```python
from build123d import *

# Parameters (mm, degrees)
SKETCH1_R                                       = 9
BOSS_EXTRUDE1_DEPTH                             = 10
SKETCH2_R                                       = 3
CUT_EXTRUDE1_DEPTH                              = 96.94790253
BOSS_EXTRUDE2_DEPTH                             = 3
SKETCH3_W                                       = 4
SKETCH3_H                                       = 8
CUT_EXTRUDE2_DEPTH                              = 97.695398029
RIB4_REACH                                      = 98.695
SKETCH5_WALL_W                                  = 220.579405852
SKETCH5_WALL_H                                  = 10
FILLET1_R                                       = 2
FILLET1_OF_MIRROR1_R                            = 2
SKETCH7_R                                       = 5
CUT_EXTRUDE3_DEPTH                              = 97.695398153
CHAMFER1_SIZE                                   = 1
CSK_FOR_M3_FLAT_HEAD_MACHINE_SCREW1_D           = 3.2
CSK_FOR_M3_FLAT_HEAD_MACHINE_SCREW1_CSINK_D     = 6.3
CSK_FOR_M3_FLAT_HEAD_MACHINE_SCREW1_CSINK_ANGLE = 90


with BuildPart() as part:
    # Sketch1 → Boss-Extrude1 (new body)
    with BuildSketch(Plane.XY):
        Circle(SKETCH1_R)
        with BuildLine():
            ThreePointArc((9, 0), (6.363961031, -6.363961031), (0, -9))
            Line((0, -9), (95, -9))
            Line((95, -9), (95, 7))
            Line((95, 7), (5.656854249, 7))
            ThreePointArc((5.656854249, 7), (8.121320344, 3.878679656), (9, 0))
        make_face()
    extrude(amount=BOSS_EXTRUDE1_DEPTH)

    # Sketch2 → Cut-Extrude1 (cut, through all)
    with BuildSketch(Plane.XY):
        Circle(SKETCH2_R)
    extrude(amount=CUT_EXTRUDE1_DEPTH, mode=Mode.SUBTRACT)

    # Sketch4 → Boss-Extrude2 (add)
    with BuildSketch(Plane(origin=(95, 0, 0), x_dir=(0, 0, -1), z_dir=(1, 0, 0))):
        with BuildLine():
            ThreePointArc((0, -14.076696831), (-5, -15), (-10, -14.076696831))
            Line((-10, -14.076696831), (-10, 12.076696831))
            ThreePointArc((-10, 12.076696831), (-5, 13), (0, 12.076696831))
            Line((0, 12.076696831), (0, -14.076696831))
        make_face()
    extrude(amount=-BOSS_EXTRUDE2_DEPTH)

    # Sketch3 → Cut-Extrude2 (cut, through all)
    with BuildSketch(Plane.XY):
        with Locations((93, -1)):
            Rectangle(SKETCH3_W, SKETCH3_H)
    extrude(amount=CUT_EXTRUDE2_DEPTH, mode=Mode.SUBTRACT)

    # Sketch5 wall → Rib4 (add, up to next)
    with BuildSketch(Plane(origin=(79.5, 8.538348415, 10), x_dir=(-0.992512099864, -0.122146353295, 0), z_dir=(0.122146353295, -0.992512099864, 0)), mode=Mode.PRIVATE) as rib4_sk1:
        with Locations((0, 5)):
            Rectangle(SKETCH5_WALL_W, SKETCH5_WALL_H)
    rib4_tool1 = extrude(rib4_sk1.sketch, amount=RIB4_REACH, mode=Mode.PRIVATE) - part.part
    rib4 = rib4_tool1.solids().sort_by_distance((79.5, 8.538348415, 10))[0]
    add(rib4)

    # Fillet1
    fillet1_edges = [part.edges().sort_by_distance(p)[0] for p in [
        (92, 11.076696831, 0),
        (92, 11.076696831, 10),
        (92, 10.07669683, 5),
        (79.500000002, 8.538348415, 0),
        (79.500000002, 8.538348415, 10),
    ]]
    fillet(fillet1_edges, radius=FILLET1_R)

    # Mirror1: Rib4 across plane
    add(rib4.mirror(Plane.ZX.offset(-1)))

    # Fillet1 of Mirror1
    fillet1_of_mirror1_edges = [part.edges().sort_by_distance(p)[0] for p in [
        (92, -13.076696831, 0),
        (92, -13.076696831, 10),
        (92, -12.07669683, 5),
        (79.500000002, -10.538348415, 0),
        (79.500000002, -10.538348415, 10),
    ]]
    fillet(fillet1_of_mirror1_edges, radius=FILLET1_OF_MIRROR1_R)

    # Sketch7 → Cut-Extrude3 (cut, through all)
    with BuildSketch(Plane.XY):
        with Locations((79.294775575, -1)):
            Circle(SKETCH7_R)
    extrude(amount=CUT_EXTRUDE3_DEPTH, mode=Mode.SUBTRACT)

    # Chamfer1
    chamfer1_edges = [part.edges().sort_by_distance(p)[0] for p in [
        (74.294775575, -1, 0),
        (74.294775575, -1, 10),
    ]]
    chamfer(chamfer1_edges, length=CHAMFER1_SIZE)

    # CSK for M3 Flat Head Machine Screw1 (through all)
    with Locations(Plane(origin=(0, 0, 0), x_dir=(-1, 0, 0), z_dir=(0, 0, -1))):
        with Locations((-17, -6)):
            CounterSinkHole(CSK_FOR_M3_FLAT_HEAD_MACHINE_SCREW1_D / 2, CSK_FOR_M3_FLAT_HEAD_MACHINE_SCREW1_CSINK_D / 2, counter_sink_angle=CSK_FOR_M3_FLAT_HEAD_MACHINE_SCREW1_CSINK_ANGLE)


solid = part.part
```
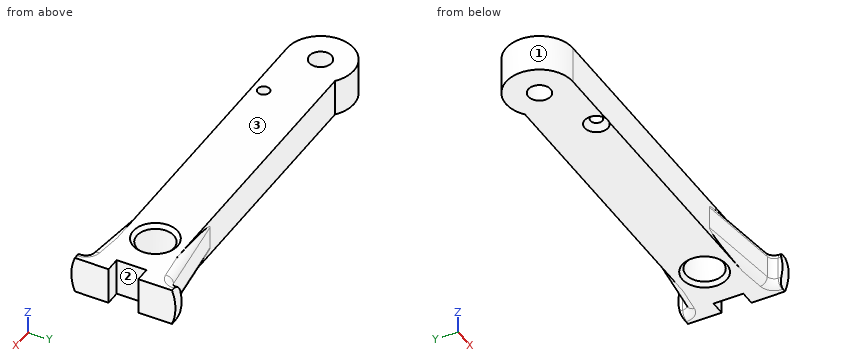
The model under review builds one solid part; all positions refer to its coordinate system, in mm. Face numbers are marked on the shaded views. Coordinates: 2 decimals unless noted, no trailing zeros. Write each loop counter-clockwise with the first axis right and the second up, starting at its lowest first coordinate (ties: lowest second). Pieces come first, ordered by that corner, then holes. Notation, with made-up numbers: (-28.5, 30.25) -> (-4.5, 30.25) arc R31 ccw to (-4.5, 62.25) -> close; hole circle Ø3 at (1, -27.5). An arc over 180 degrees is marked (long way). One line per item, written item: value. Start each with the question number.
Q1. To check wall thickness, follow probe 1 along Y at (x, z) = (17, 5.5); probe 2 along Y at (x, z) = (24, 1); probe 3 along X at (y, z) = (-1, 0.5). State the ranges of each line that lie inside material, in increasing order.
Q2. Add section B-B, the plane z = 3.5. Give the boundary of the cut face in (x, y).
Q3. The part is to be moulded in two halves that separate along X. For the marked faces 1, 2 and 3, say which applies: +X half, -X half, draft (parallel to the pull), parting line (faces both ways), or undercut.
Q4. Clearance check with flat-ended pins moving along their axes: P1, Ø3.5, axis at x = 17, y = -6, coming from the +Z side; P2, Ø0.6, axis at y = -14.5, z = 5, coming from the -X side; P3, Ø4, axis at y = 0, z = 7.5, coming from the +X side; P4, Ø1.5, axis at x = 19.5, z = 6.5, coming from the +Y side. State where each tip first meets the part, or that it passes through.
Q5. Add section C-C, the plane y = -1. Give the boundary of the cut face in (x, z), then the cut area to 3 significant figures.
Q6. Add section A-A, the plane x = 17. Give the boundary of the cut face in (y, z).
Response:
1. probe 1: -9 to -7.6, -4.4 to 7
1. probe 2: -9 to 7
1. probe 3: -8.94 to -2.83, 2.83 to 73.79, 84.79 to 91
2. outline: (0, -9) -> (67, -9) -> (90.24, -11.86) arc R2 cw to (92, -13.85) -> (92, -14.92) -> (95, -14.92) -> (95, -5) -> (91, -5) -> (91, 3) -> (95, 3) -> (95, 12.92) -> (92, 12.92) -> (92, 11.85) arc R2 cw to (90.24, 9.86) -> (67, 7) -> (5.66, 7) arc R9 ccw (long way) to start; hole circle Ø6 at (0, 0); hole circle Ø3.2 at (17, -6); hole circle Ø10 at (79.29, -1)
3. face 1: undercut
3. face 2: +X half
3. face 3: draft
4. P1: z = 10
4. P2: x = 92
4. P3: x = 91
4. P4: y = 7
5. outline: (-8.94, 0) -> (-2.83, 0) -> (-2.83, 10) -> (-8.94, 10) -> close; (2.83, 0) -> (73.29, 0) -> (74.29, 1) -> (74.29, 9) -> (73.29, 10) -> (2.83, 10) -> close; (84.29, 1) -> (85.29, 0) -> (91, 0) -> (91, 10) -> (85.29, 10) -> (84.29, 9) -> close
5. area: 841 mm²
6. outline: (-9, 0.15) -> (-7.6, 1.55) -> (-7.6, 10) -> (-9, 10) -> close; (-4.4, 1.55) -> (-2.85, 0) -> (7, 0) -> (7, 10) -> (-4.4, 10) -> close
